from build123d import *

# Parameters (mm, degrees)
SKETCH1_W           = 24
SKETCH1_H           = 15.2
BOSS_EXTRUDE1_DEPTH = 10
SKETCH3_R           = 1.75
CUT_EXTRUDE1_DEPTH  = 10
BOSS_EXTRUDE2_DEPTH = 12


with BuildPart() as part:
    # Sketch1 → Boss-Extrude1 (new body)
    with BuildSketch(Plane(origin=(0, 0, 0), x_dir=(1, 0, 0), z_dir=(0, 1, 0))):
        Rectangle(SKETCH1_W, SKETCH1_H)
    extrude(amount=BOSS_EXTRUDE1_DEPTH)

    # Sketch3 → Cut-Extrude1 (cut)
    with BuildSketch(Plane(origin=(0, 10, 0), x_dir=(1, 0, 0), z_dir=(0, 1, 0))):
        with Locations(Location((5, -0.1, 0), (0, 0, 270))):
            Circle(SKETCH3_R)
    extrude(amount=-CUT_EXTRUDE1_DEPTH, mode=Mode.SUBTRACT)

    # Sketch4 → Boss-Extrude2 (add)
    with BuildSketch(Plane(origin=(0, 0, 0), x_dir=(-1, 0, 0), z_dir=(0, -1, 0))):
        Polygon((12, -9.6), (12, -7.6), (-12, -7.6), (-12, 7.6), (12, 7.6), (12, 9.6), (-14, 9.6), (-14, -9.6), align=None)
    extrude(amount=-BOSS_EXTRUDE2_DEPTH)


solid = part.part
The listing builds one solid part. Answer for the finished solid, in the listing's coordinates (mm). A direction names the side the tool comes from. Give positions to 0.01 mm unless a question says otherwise; leave off trailing zeros. Write each loop counter-clockwise with the first axis right and the second up, starting at its lowest first coordinate (ties: lowest second). Pieces come first, ordered by that corner, then holes. Notation, with made-up numbers: (42.25, 47.5) - (100.25, 47.5) arc R22 cw to (100.25, 71.5) - close; hole circle Ø6 at (56.25, 46). An arc over 180 degrees is marked (long way). One line per question, with ' | ' between items. Start each with the question number.
1. Straight lines are drawn through the part: line 1 (X direction, y = 6.5, z = 0.1); line 2 (Z direction, x = 4, y = 10.75); line 3 (Y direction, x = 1.75, z = -0.5). For each, find the intervals that lie inside material, in ascending order.
2. Determine the mould class of faces 1 (the face through (1, 6, -9.6)), 2 (the face through (-12, 6, 0)), 3 (the face through (0, 11, -7.6)), 4 (the face through (12, 11, 0)) for opening direction Z: +Z half, -Z half, draft (parallel to the pull), parting line (faces both ways), or undercut.
3. For faces 5 (the face through (4, 12, 8)), 6 (the face through (0, 10, 0)), determine the directions among +Z, -Z, +X, -X, +Y, -Y from which every point of the face is accessible in a straight line to the end or side of a thin tool.
4. Given P1, Ø0.6, axis at y = 11, z = 4, coming from the -X side; P2, Ø1.5, axis at x = -8, z = 3.5, coming from the +Y side, each flat-ended and moving along its own axis, determine where each tip first touches the part or whether it passes through.
5. Section C-C, the plane y = 2 is taken. Determine the outline of the cut face in (x, z).
6. Section A-A, the plane x = 5 is taken. Determine the outline of the cut face in (y, z), then the cut area to 3 significant figures.
7. Section B-B, the plane z = 0.1 is taken. Determine the outline of the cut face in (x, y), then the cut area to 3 significant figures.
8. Section D-D, the plane x = -1.25 is taken. Determine the outline of the cut face in (y, z), then the cut area to 3 significant figures.
Result:
1) line 1: x = -12 to 3.25, 6.75 to 14 | line 2: z = -9.6 to -7.6, 7.6 to 9.6 | line 3: y = 0 to 10
2) face 1: -Z half | face 2: draft | face 3: undercut | face 4: undercut
3) face 5: +Z, -Z, +X, -X, +Y | face 6: -X, +Y
4) P1: stops at x = 12 | P2: stops at y = 10
5) outline: (-12, -9.6) - (14, -9.6) - (14, 9.6) - (-12, 9.6) - close; hole circle Ø3.5 at (5, 0.1)
6) outline: (0, -9.6) - (12, -9.6) - (12, -7.6) - (10, -7.6) - (10, -1.65) - (0, -1.65) - close; (0, 1.85) - (10, 1.85) - (10, 7.6) - (12, 7.6) - (12, 9.6) - (0, 9.6) - close | area: 165 mm2
7) outline: (-12, 0) - (3.25, 0) - (3.25, 10) - (-12, 10) - close; (6.75, 0) - (14, 0) - (14, 12) - (12, 12) - (12, 10) - (6.75, 10) - close | area: 229 mm2
8) outline: (0, -9.6) - (12, -9.6) - (12, -7.6) - (10, -7.6) - (10, 7.6) - (12, 7.6) - (12, 9.6) - (0, 9.6) - close | area: 200 mm2
